Study the drawing (mm; zero at the part's minimum x, y, z) and answer. A direction names the side the tool comes from. Coordinates: 2 decimals unless noted, no trailing zeros. Loops run counter-clockwise (first coordinate to the right, second up) from the corner with the lowest first, then second, coordinate; pieces in that order, holes last. Notation, with made-up numbers: (-20, 10.5) -> (23, 10.5) arc R22 cw to (23, 31.5) -> close; hole circle Ø1 at (-21.75, 50). An arc over 180 degrees is marked (long way). One line per question, with ' | ' between items.
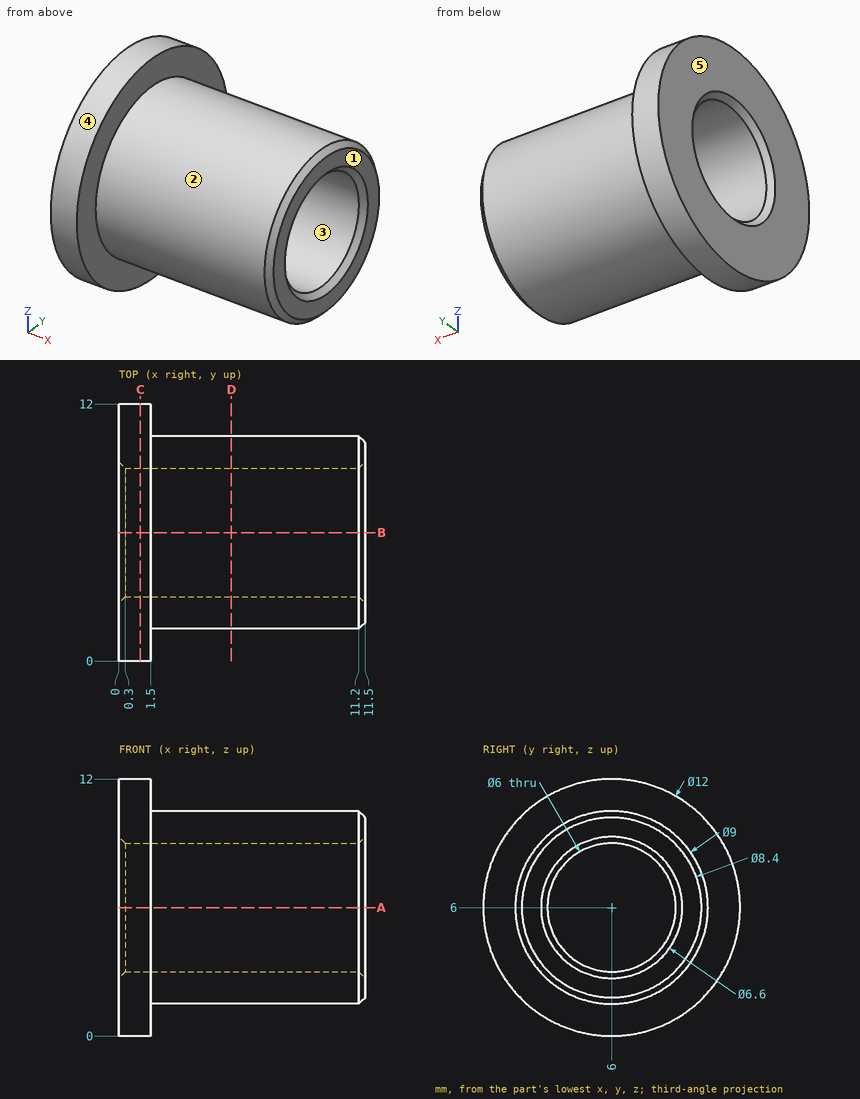
1) Find section C-C (x = 1). Write down the section's boundary in (y, z).
Check values:
outline: circle Ø12 at (6, 6); hole circle Ø6 at (6, 6)
2) Find section A-A (z = 6). Write down the section's boundary in (x, y), plus the area to 3 significant figures.
Check values:
outline: (0, 0) -> (1.5, 0) -> (1.5, 1.5) -> (11.2, 1.5) -> (11.5, 1.8) -> (11.5, 2.7) -> (11.2, 3) -> (0.3, 3) -> (0, 2.7) -> close; (0, 9.3) -> (0.3, 9) -> (11.2, 9) -> (11.5, 9.3) -> (11.5, 10.2) -> (11.2, 10.5) -> (1.5, 10.5) -> (1.5, 12) -> (0, 12) -> close | area: 38.7 mm^2
3) The mould has two halves that part along Y. Classify the marked faces 3, 4 and 5: released by +Y, released by -Y, zero draft, split by the parting line, or undercut.
Check values:
face 3: undercut | face 4: split by the parting line | face 5: zero draft
4) Find section D-D (x = 5.25). Write down the section's boundary in (y, z), plus the area to 3 significant figures.
Check values:
outline: circle Ø9 at (6, 6); hole circle Ø6 at (6, 6) | area: 35.3 mm^2
5) Flat-ended cylindrical pins translate along their axes: pin 1 (6 mm diameter, centred on x = 8, y = 3, fed in from +Z); pin 2 (2 mm diameter, centred on x = 5, z = 7, fed in from -Y); pin 3 (1.5 mm diameter, centred on x = 1.5, z = 8.5, fed in from +Y). Find the tip coordinate at first contact, or state that the pin passes through.
Check values:
pin 1: stops at z = 10.5 | pin 2: stops at y = 1.5 | pin 3: stops at y = 11.74
6) For the marked faces 1 and 2, determine the directions among +Z, -Z, +X, -X, +Y, -Y from which every point of the face is accessible in a straight line to the end or side of a thin tool.
Check values:
face 1: +Z, -Z, +X, +Y, -Y | face 2: +X
7) Find the intervals of material crossed by line 1 along Z through (x, y) = (7.5, 6); line 2 along X through (y, z) = (2, 9.5); line 3 along Y through (x, z) = (10, 4.75), in increasing order.
Check values:
line 1: z = 1.5 to 3, 9 to 10.5 | line 2: x = 0 to 1.5 | line 3: y = 1.68 to 3.27, 8.73 to 10.32
